Input: part model. Units: mm. Frame: model coordinates. A direction names the side the tool comes from. Give positions to 0.01 mm unless a question says otherwise; leave off trailing zeros. Loops run counter-clockwise (first coordinate to the right, second up) from the corner with the lowest first, then second, coordinate; pieces in that order, holes last. Notation, with made-up numbers: (40.5, -26) -> (83.5, -26) arc R14 ccw to (83.5, -4) -> close; hole circle Ø2 at (-19, 51.5). An arc over 180 degrees is marked (long way). Answer as a JSON object with one key per item and string values. Group by question number.
```python
from build123d import *

# Parameters (mm, degrees)
SKETCH_1_R      = 1.6
EXTRUDE_1_DEPTH = 3
SKETCH_2_W      = 30
SKETCH_2_H      = 5
EXTRUDE_2_DEPTH = 5.5
FILLET_1_R      = 10


with BuildPart() as part:
    # 草图1 → 凸台-拉伸1 (new body)
    with BuildSketch(Plane(origin=(0, 0, 0), x_dir=(1, 0, 0), z_dir=(0, 1, 0))):
        with BuildLine():
            Line((-5, 0), (-5, -9.5))
            Line((-5, -9.5), (5, -9.5))
            Line((5, -9.5), (5, 0))
            ThreePointArc((5, 0), (0, 5), (-5, 0))
        make_face()
        with Locations(Location((0, 0, 0), (0, 0, 270))):
            Circle(SKETCH_1_R, mode=Mode.SUBTRACT)
    extrude(amount=EXTRUDE_1_DEPTH)

    # 草图2 → 凸台-拉伸2 (add)
    with BuildSketch(Plane(origin=(0, 3, 0), x_dir=(1, 0, 0), z_dir=(0, 1, 0))):
        with Locations((0, -12)):
            Rectangle(SKETCH_2_W, SKETCH_2_H)
    extrude(amount=-EXTRUDE_2_DEPTH)

    # 圆角1
    # the kernel refuses this fillet: 10 mm, written as the material it adds along each edge
    with BuildSketch(Plane(origin=(-5, 0, 9.5), x_dir=(-1, 0, 0), z_dir=(0, 1, 0))) as fillet_1_piece_1:
        with BuildLine():
            CenterArc((9.991664351, -10), FILLET_1_R, 90, 88.089786828)
            Line((-0.00277855, -9.666666667), (-1.00222284, -9.633333333))
            ThreePointArc((-1.00222284, -9.633333333), (-1, -9.5), (-1, 0))
            Line((-1, 0), (0, 1))
            Line((0, 1), (9.991664351, 1))
            Line((9.991664351, 1), (9.991664351, 0))
        make_face()
    extrude(amount=3)
    with BuildSketch(Plane(origin=(5, 0, 9.5), x_dir=(1, 0, 0), z_dir=(0, 1, 0))) as fillet_1_piece_2:
        with BuildLine():
            CenterArc((9.991664351, 10), FILLET_1_R, 181.910213172, 88.089786828)
            Line((-0.00277855, 9.666666667), (-1.00222284, 9.633333333))
            ThreePointArc((-1.00222284, 9.633333333), (-1, 9.5), (-1, 0))
            Line((-1, 0), (0, -1))
            Line((0, -1), (9.991664351, -1))
            Line((9.991664351, -1), (9.991664351, 0))
        make_face()
    extrude(amount=3)


solid = part.part
```
Q1. Pull-direction query (X, two-part tool) for faces 1 (the face through (-0.97, 1.48, -1.27)), 2 (the face through (0, 1, -5)), 3 (the face through (-15, 0, 12)); classes: +X half, -X half, draft (parallel to the pull), parting line (faces both ways), or undercut.
Q2. Section C-C on z = -3. Return the cut outline in (x, y), then the cut area to 3 significant figures.
Q3. Ray query, probe 1 along X at (y, z) = (1.35, 0); probe 2 along Z at (x, y) = (-11.25, -1.75); probe 3 along X at (y, z) = (1.3, -0.5). Return the intervals inside material, ascending.
Q4. Section A-A on x = 0. Return the cut outline in (y, z), then the cut area to 3 significant figures.
Q5. Set-up query: faces 4 (the face through (0, 3, 7)), 5 (the face through (0, 0, 4)). Return all of +Z, -Z, +X, -X, +Y, -Y with unobstructed straight access to the full face (end or side cutting, diameter ignored); none if empty.
Q6. Section D-D on x = -3. Return the cut outline in (y, z), then the cut area to 3 significant figures.
Q7. Pin query (flat end, axial travel): pin 1 Ø3.5 at (x, z) = (0, 0) entering from +Y; pin 2 Ø1.5 at (x, y) = (-2.5, 2) entering from -Z; pin 3 Ø6 at (x, z) = (-6.5, -2.5) entering from -Y; pin 4 Ø1.6 at (x, y) = (-6.5, -1) entering from -Z. Return the tip coordinate at first contact, or that it passes through.
Numbers:
{
 "1": {"face 1": "undercut", "face 2": "parting line", "face 3": "-X half"},
 "2": {"outline": "(-4, 0) -> (4, 0) -> (4, 3) -> (-4, 3) -> close", "area": "24.0 mm²"},
 "3": {"probe 1": "x = -5 to -1.6, 1.6 to 5", "probe 2": "z = 9.5 to 14.5", "probe 3": "x = -4.97 to -1.52, 1.52 to 4.97"},
 "4": {"outline": "(-2.5, 9.5) -> (0, 9.5) -> (0, 1.6) -> (3, 1.6) -> (3, 14.5) -> (-2.5, 14.5) -> close; (0, -5) -> (3, -5) -> (3, -1.6) -> (0, -1.6) -> close", "area": "61.4 mm²"},
 "5": {"face 4": "+Z, -Z, +X, -X, +Y", "face 5": "-Z, +X, -X, -Y"},
 "6": {"outline": "(-2.5, 9.5) -> (0, 9.5) -> (0, -4) -> (3, -4) -> (3, 14.5) -> (-2.5, 14.5) -> close", "area": "68.0 mm²"},
 "7": {"pin 1": "stops at y = 3", "pin 2": "stops at z = -4.68", "pin 3": "stops at y = 0", "pin 4": "stops at z = 9.5"}
}
